```python
from build123d import *

# Parameters (mm, degrees)
EXTRUDE003_DEPTH                          = 2.658721
EXTRUDE003_ONTO_SKETCH010_ROLL_ANGLE      = 90
EXTRUDE003_ONTO_SKETCH010_PLACEMENT_ANGLE = 45
EXTRUDE002_DEPTH                          = 2.65
EXTRUDE001_DEPTH                          = 2.65
EXTRUDE_DEPTH                             = 45
POCKET_DEPTH                              = 30.001
POCKET001_DEPTH                           = 30.001019
SKETCH003_R                               = 1.55
POCKET002_DEPTH                           = 16
SKETCH005_R                               = 3.1
POCKET003_DEPTH                           = 5
SKETCH006_R                               = 1.55
POCKET004_DEPTH                           = 16
SKETCH008_R                               = 3.1
POCKET005_DEPTH                           = 5
SKETCH009_R                               = 1.55
POCKET006_DEPTH                           = 10
FILLET_R                                  = 0.9


with BuildPart() as extrude003:
    # Sketch010 as drawn → Extrude003 (new)
    with BuildSketch(Plane.XY):
        Polygon((3.262029, 22.5), (1.631015, 25.325), (-13.368985, 25.325), (-13.368985, 19.675), (1.631015, 19.675), align=None)
    extrude(amount=-EXTRUDE003_DEPTH)


with BuildPart() as extrude003_1:
    # Extrude003 onto Sketch010 roll: moved
    add(extrude003.part.rotate(Axis((0, 0, 0), (1, 0, 0)), EXTRUDE003_ONTO_SKETCH010_ROLL_ANGLE))


with BuildPart() as extrude003_2:
    # Extrude003 onto Sketch010 placement: moved
    add(extrude003_1.part.moved(Location((11.464466, -11.464466, 0))).rotate(Axis((11.464466, -11.464466, 0), (0, 0, 1)), EXTRUDE003_ONTO_SKETCH010_PLACEMENT_ANGLE))


with BuildPart() as extrude003_3:
    # Extrude003 placement: moved
    add(extrude003_2.part.moved(Location((-2.5, 2.5, 0))))


with BuildPart() as extrude002:
    # Sketch007 → Extrude002 (new body)
    with BuildSketch(Plane(origin=(0, 0, 0), x_dir=(1, 0, 0), z_dir=(0, 0, -1))):
        Polygon((0, -7.737971), (-2.825, -9.368985), (-2.825, -15), (2.825, -15), (2.825, -9.368985), align=None)
    extrude(amount=-EXTRUDE002_DEPTH)


with BuildPart() as extrude002_1:
    # Extrude002 placement: moved
    add(extrude002.part.moved(Location((0, 0, 14))))


with BuildPart() as extrude001:
    # Sketch004 → Extrude001 (new body)
    with BuildSketch(Plane.XY.offset(45)):
        Polygon((-7.737971, 0), (-9.368985, 2.825), (-15, 2.825), (-15, -2.825), (-9.368985, -2.825), align=None)
    extrude(amount=-EXTRUDE001_DEPTH)


with BuildPart() as extrude001_1:
    # Extrude001 placement: moved
    add(extrude001.part.moved(Location((0, 0, -14))))


with BuildPart() as fillet_body:
    # Sketch → Extrude (new body)
    with BuildSketch(Plane.XY):
        with BuildLine():
            Line((15, -7.928932), (7.928932, -15))
            Line((7.928932, -15), (-9, -15))
            ThreePointArc((-15, -9), (-13.242641, -13.242641), (-9, -15))
            Line((-15, -9), (-15, 9))
            ThreePointArc((-9, 15), (-13.242641, 13.242641), (-15, 9))
            Line((-9, 15), (9, 15))
            ThreePointArc((15, 9), (13.242641, 13.242641), (9, 15))
            Line((15, 9), (15, -7.928932))
        make_face()
    extrude(amount=EXTRUDE_DEPTH)

    # Sketch001 → Pocket (cut, through all)
    with BuildSketch(Plane(origin=(-15, 0, 0), x_dir=(0, -1, 0), z_dir=(-1, 0, 0))):
        with BuildLine():
            Line((9, 0), (15, 0))
            Line((15, 0), (15, 6))
            ThreePointArc((9, 0), (13.242641, 1.757359), (15, 6))
        make_face()
        with BuildLine():
            ThreePointArc((-7.640803, 9.625), (7.65, 10), (-7.640803, 10.375))
            Line((-7.640803, 10.375), (-15.640803, 10.375))
            Line((-15.640803, 10.375), (-15.640803, 9.625))
            Line((-15.640803, 9.625), (-7.640803, 9.625))
        make_face()
    extrude(amount=-POCKET_DEPTH, mode=Mode.SUBTRACT)

    # Sketch002 → Pocket001 (cut, through all)
    with BuildSketch(Plane(origin=(0, 15, 0), x_dir=(-1, 0, 0), z_dir=(0, 1, 0))):
        with BuildLine():
            ThreePointArc((-9, 45), (-13.242641, 43.242641), (-15, 39))
            Line((-15, 39), (-15, 45))
            Line((-15, 45), (-9, 45))
        make_face()
        with BuildLine():
            ThreePointArc((7.640803, 35.375), (-7.65, 35), (7.640803, 34.625))
            Line((15.640803, 34.625), (7.640803, 34.625))
            Line((15.640803, 35.375), (15.640803, 34.625))
            Line((7.640803, 35.375), (15.640803, 35.375))
        make_face()
    extrude(amount=-POCKET001_DEPTH, mode=Mode.SUBTRACT)

    # Sketch003 → Pocket002 (cut)
    with BuildSketch(Plane.XY.offset(45)):
        with Locations((-11, 0)):
            Circle(SKETCH003_R)
    extrude(amount=-POCKET002_DEPTH, mode=Mode.SUBTRACT)

    # Cut: cut Extrude001
    add(extrude001_1.part, mode=Mode.SUBTRACT)

    # Sketch005 → Pocket003 (cut)
    with BuildSketch(Plane.XY.offset(45)):
        with Locations((-11, 0)):
            Circle(SKETCH005_R)
    extrude(amount=-POCKET003_DEPTH, mode=Mode.SUBTRACT)

    # Sketch006 → Pocket004 (cut)
    with BuildSketch(Plane(origin=(0, 0, 0), x_dir=(1, 0, 0), z_dir=(0, 0, -1))):
        with Locations((0, -11)):
            Circle(SKETCH006_R)
    extrude(amount=-POCKET004_DEPTH, mode=Mode.SUBTRACT)

    # Cut001: cut Extrude002
    add(extrude002_1.part, mode=Mode.SUBTRACT)

    # Sketch008 → Pocket005 (cut)
    with BuildSketch(Plane(origin=(0, 0, 0), x_dir=(1, 0, 0), z_dir=(0, 0, -1))):
        with Locations((0, -11)):
            Circle(SKETCH008_R)
    extrude(amount=-POCKET005_DEPTH, mode=Mode.SUBTRACT)

    # Sketch009 → Pocket006 (cut)
    with BuildSketch(Plane(origin=(11.464466, -11.464466, 0), x_dir=(0.707107, 0.707107, 0), z_dir=(0.707107, -0.707107, 0))):
        with Locations((0, 22.5)):
            Circle(SKETCH009_R)
    extrude(amount=-POCKET006_DEPTH, mode=Mode.SUBTRACT)

    # Cut002: cut Extrude003
    add(extrude003_3.part, mode=Mode.SUBTRACT)

    # Fillet
    fillet_edges = [fillet_body.edges().sort_by_distance(p)[0] for p in [
        (-15, 8.320402, 10.375),
        (-15, -7.65, 10),
        (-15, 8.320402, 9.625),
        (-15, 0, 34.625),
        (-15, 0, 28.35),
        (-15, -2.825, 29.675),
        (-15, 0, 31),
        (-15, 2.825, 29.675),
        (-15, 0, 35.375),
    ]]
    fillet(fillet_edges, radius=FILLET_R)


solid = fillet_body.part
```
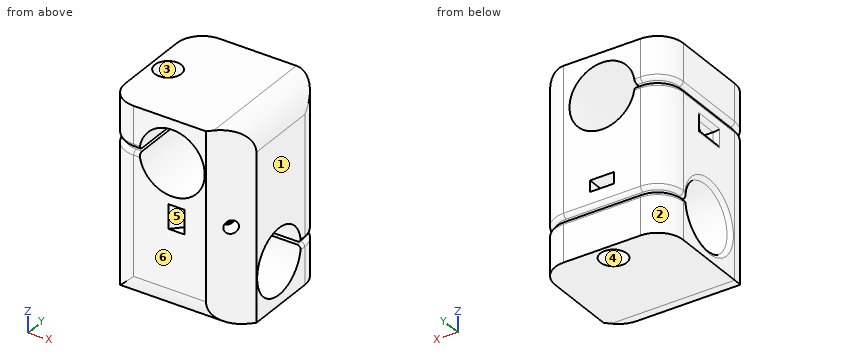
Could you check a few things on this model? Use its own coordinates, in mm. Face numbers are marked on the shaded views. A direction names the side the tool comes from. Coordinates: 2 decimals unless noted, no trailing zeros. Write each loop counter-clockwise with the first axis right and the second up, starting at its lowest first coordinate (ties: lowest second). Pieces come first, ordered by that corner, then holes. Notation, with made-up numbers: (58.25, -7) -> (67.25, -7) arc R19 ccw to (67.25, -2) -> close; hole circle Ø3 at (12.25, 30.5). An arc over 180 degrees is marked (long way). Write item = value, one per line. Start each with the question number.
(1) Will these pins go through, and if not, where does the flat tip stop? pin 1 (5 mm diameter, centred on x = 0, y = 11, fed in from -Z); pin 2 (2 mm diameter, centred on x = -11.5, z = 29.5, fed in from +Y); pin 3 (8 mm diameter, centred on y = 10, z = 17.5, fed in from -X); pin 4 (5 mm diameter, centred on x = -11, y = 0, fed in from +Z).
(2) Which directions (+Z, -Z, +X, -X, +Y, -Y) give clear straight access to the entire face, cutting with the end or side of a thin tool? Please do the marked faces 4, 5 and 6.
(3) I want a section at B-B (y = 11). Give the number of separate pieces and of enclosed holes in the cut face, plus the area to 3 significant figures.
(4) I need wall thicknesses on line 1 (Z direction, x = -13, y = -3) (3 decimals); line 2 (Z direction, x = 3, y = -6); line 3 (X direction, y = -11, z = 25). Which ranges of each line are inside material? Lowest first, please. Write a range as [from, to].
(5) We'd pull the mould along Y, two halves only. Please class the marked faces 1, 2 and 3: released by +Y, released by -Y, zero draft, split by the parting line, or undercut.
(6) I want a section at A-A (x = -4). Please give me the cut outline in (y, z) (3 decimals).
Result set:
q1.pin_1 = 5
q1.pin_2 = 14.81
q1.pin_3 = -15
q1.pin_4 = 40
q2.face_4 = -Z
q2.face_5 = none
q2.face_6 = +Z, -Z, +X, -X, -Y
q3.separate_pieces = 3
q3.enclosed_holes = 0
q3.area = 1,030 mm2
q4.line_1 = [0, 2.963], [17.037, 34.625], [35.375, 45]
q4.line_2 = [0, 5.25], [14.75, 27.96], [42.04, 45]
q4.line_3 = [-14.66, 3.17], [6.93, 11.93]
q5.face_1 = zero draft
q5.face_2 = released by +Y
q5.face_3 = undercut
q6.outline = (-15, 6) arc R6 ccw to (-9, 0) -> (15, 0) -> (15, 8.725) arc R0.9 ccw to (14.1, 9.625) -> (7.641, 9.625) arc R7.65 cw (long way) to (7.641, 10.375) -> (14.1, 10.375) arc R0.9 ccw to (15, 11.275) -> (15, 28.479) -> (-15, 28.479) -> close; (-15, 41.521) -> (15, 41.521) -> (15, 45) -> (-15, 45) -> close
